Could you check a few things on this model? Use its own coordinates, in mm. A direction names the side the tool comes from. Round coordinates to 2 decimals unless told otherwise and drop trailing zeros. Write each loop counter-clockwise with the first axis right and the second up, starting at its lowest first coordinate (ties: lowest second). Pieces come first, ordered by that corner, then holes. Notation, with made-up numbers: (-9, -21) - (42, -21) arc R27 cw to (42, -2) - close; hole circle Ø5 at (76.25, 31). An arc over 180 degrees is marked (long way). Put each result on its own line as item: value.
from build123d import *

# Parameters (mm, degrees)
F0_R     = 11
F0_R_2   = 4
F1_DEPTH = 7
F2_SIZE  = 0.508
F3_R     = 9.5
F3_R_2   = 6
F4_DEPTH = 0.254
F5_R     = 9.5
F5_R_2   = 6
F6_DEPTH = 0.254


with BuildPart() as f1:
    # F0 (on Front) → F1 (new body)
    with BuildSketch(Plane.XZ):
        Circle(F0_R)
        Circle(F0_R_2, mode=Mode.SUBTRACT)
    extrude(amount=F1_DEPTH)

    # F2
    f2_edges = [f1.edges().sort_by_distance(p)[0] for p in [
        (11, -3.5, 0),
        (-11, 0, 0),
        (-11, -7, 0),
        (4, -3.5, 0),
        (-4, 0, 0),
        (-4, -7, 0),
    ]]
    chamfer(f2_edges, length=F2_SIZE)

    # F3 (on face) → F4 (cut)
    with BuildSketch(Plane(origin=(0, 0, 0), x_dir=(-1, 0, 0), z_dir=(0, 1, 0))):
        Circle(F3_R)
        Circle(F3_R_2, mode=Mode.SUBTRACT)
    extrude(amount=-F4_DEPTH, mode=Mode.SUBTRACT)

    # F5 (on face) → F6 (cut)
    with BuildSketch(Plane.XZ.offset(7)):
        Circle(F5_R)
        Circle(F5_R_2, mode=Mode.SUBTRACT)
    extrude(amount=-F6_DEPTH, mode=Mode.SUBTRACT)


solid = f1.part
(1) Please list where these lines run through material, in increasing order: probe 1 along Z at (x, y) = (0, -5); probe 2 along Z at (x, y) = (0, -0.1); probe 3 along X at (y, z) = (-4.75, -2). Write a range as from..to.
Values found:
probe 1: z = -11..-4, 4..11
probe 2: z = -10.59..-9.5, -6..-4.41, 4.41..6, 9.5..10.59
probe 3: x = -10.82..-3.46, 3.46..10.82
(2) For faces 1 (the face through (0.1, -0.254, -6.2)), 2 (the face through (-1.4, -7, 4.5)), which set-ups out of +Z, -Z, +X, -X, +Y, -Y let a thin tool reach every point of the face, with its end or its side?
Values found:
face 1: +Y
face 2: +Z, -Z, +X, -X, -Y
(3) I'm going to push flat-ended pins straight in: pin 1 (1 mm diameter, centred on y = -5.5, z = -6, fed in from -X); pin 2 (1.5 mm diameter, centred on y = -2, z = -3, fed in from -X); pin 3 (1.5 mm diameter, centred on y = -1.5, z = -1.5, fed in from +X). Where does each tip first touch, or does it pass through?
Values found:
pin 1: stops at x = -9.53
pin 2: stops at x = -10.77
pin 3: stops at x = 10.97
(4) If we mould it in two halves opening along X, with no side actions, what happens to faces 3 (the face through (-2.38, -3.46, -10.74)), 4 (the face through (-1.4, 0, 4.5)), 5 (the face through (-0.867, -3.458, -3.905)), 6 (the face through (-0.1, -6.746, -6.2))? For each: pulls with the +X half, pulls with the -X half, needs draft (parallel to the pull), parting line crosses it, or undercut.
Values found:
face 3: parting line crosses it
face 4: needs draft
face 5: undercut
face 6: undercut
(5) Imagine slicing it at C-C, the plane y = -2. List the corners of the cut face in (x, z) for me, then the cut area to 3 significant figures.
Values found:
outline: circle Ø22 at (0, 0); hole circle Ø8 at (0, 0)
area: 330 mm^2
